Verification items for the finished model (mm, model axes). A direction names the side the tool comes from. Round coordinates to 2 decimals unless told otherwise and drop trailing zeros. Write each loop counter-clockwise with the first axis right and the second up, starting at its lowest first coordinate (ties: lowest second). Pieces come first, ordered by that corner, then holes. Notation, with made-up numbers: M 39,-5 L 85,-5 A30 cw 85,27 Z; hole C 61,41.5 d2. An arc over 180 degrees is marked long. One line per item, written item: value. Start each with the question number.
Item 1: Section check A-A, the plane y = 44. Record the cut outline in (x, z), then the cut area to 3 significant figures.
Item 2: Section check D-D, the plane x = 0.5. Record the cut outline in (y, z).
Item 3: Section check B-B, the plane x = 17.5. Record the cut outline in (y, z).
Item 4: Thickness scan on probe 1 along Z at (x, y) = (17.5, -17.25); probe 2 along X at (y, z) = (-18, 5.25); probe 3 along Z at (x, y) = (-9, 40). Record the ranges inside material, lowest first. Write a range as from..to.
Item 5: Draft check along X on faces 1 (the face through (17, -8, 2)), 2 (the face through (-15, -32, 2)), 3 (the face through (0, -2, 3.1)). Enter one of: +X half, -X half, draft (parallel to the pull), parting line (faces both ways), or undercut.
Item 6: Tool access check on faces 4 (the face through (-7, 35, 2)), 5 (the face through (18.655, -21.605, 2.021)), 6 (the face through (0, -2, 0)), 7 (the face through (-18, -8, 2)), 8 (the face through (15.85, 44, 2)). Record the directions out of +Z, -Z, +X, -X, +Y, -Y that give a thin tool (end or side, any length) a straight path to the whole face; none if there is none.
Item 7: Gauge pin test, flat ends, axial feed: pin 1 (0.9 mm diameter, centred on y = -11, z = 1.5, fed in from -X); pin 2 (2.5 mm diameter, centred on y = 46.5, z = 1.5, fed in from -X); pin 3 (1.6 mm diameter, centred on y = -10, z = 1, fed in from +X); pin 4 (2 mm diameter, centred on x = -17.5, z = 8.6, fed in from +Y). Record the tip position at first contact, or that the pin passes through.
Item 8: Section check C-C, the plane z = 8.6. Record the cut outline in (x, y), then the cut area to 3 significant figures.
from build123d import *

# Parameters (mm, degrees)
F0_W      = 3.95
F0_H      = 17.6
F0_W_2    = 3.8
F1_DEPTH  = 3.1
F2_W      = 40
F2_H      = 24
F3_DEPTH  = 1.5
F5_DEPTH  = 1.5
F6_W      = 5
F6_H      = 15
F7_DEPTH  = 8
F8_W      = 5
F8_H      = 6
F9_DEPTH  = 4.601
F10_R     = 1.25
F11_DEPTH = 15
F12_R     = 1.25
F13_DEPTH = 15


with BuildPart() as f1:
    # F0 (on Top) → F1 (new body)
    with BuildSketch(Plane.XY):
        with Locations((0.025, 43.8)):
            Rectangle(F0_W, F0_H)
        with Locations((-13.95, 43.8)):
            Rectangle(F0_W_2, F0_H)
        with Locations((13.95, 43.8)):
            Rectangle(F0_W_2, F0_H)
        Polygon((20, -35), (20, 35), (15.85, 35), (12.05, 35), (2, 35), (-1.95, 35), (-12.05, 35), (-15.85, 35), (-20, 35), (-20, -35), align=None)
    extrude(amount=F1_DEPTH)

    # F2 (on face) → F3 (join)
    with BuildSketch(Plane.XY.offset(3.1)):
        with Locations((0, 42)):
            Rectangle(F2_W, F2_H)
    extrude(amount=F3_DEPTH)

    # F4 (on face) → F5 (join)
    with BuildSketch(Plane(origin=(0, 0, 0), x_dir=(1, 0, 0), z_dir=(0, 0, -1))):
        Polygon((20.048024, -30), (20, -30), (20, -35), (15.85, -35), (15.85, -52.6), (12.05, -52.6), (12.05, -35), (2, -35), (2, -52.6), (-1.95, -52.6), (-1.95, -35), (-12.05, -35), (-12.05, -52.6), (-15.85, -52.6), (-15.85, -35), (-20, -35), (-20, -54), (20.048024, -54), align=None)
        Polygon((20, -30), (-20, -30), (-20, -35), (-15.85, -35), (-15.85, -52.6), (-12.05, -52.6), (-12.05, -35), (-1.95, -35), (-1.95, -52.6), (2, -52.6), (2, -35), (12.05, -35), (12.05, -52.6), (15.85, -52.6), (15.85, -35), (20, -35), align=None)
    extrude(amount=F5_DEPTH)

    # F6 (on face) → F7 (join)
    with BuildSketch(Plane.XY.offset(3.1)):
        with Locations((17.5, -21.5)):
            Rectangle(F6_W, F6_H)
        with Locations((-17.5, -21.5)):
            Rectangle(F6_W, F6_H)
    extrude(amount=F7_DEPTH)

    # F8 (on face) → F9 (cut, through all)
    with BuildSketch(Plane.XY.offset(3.1)):
        with Locations((17.5, -32)):
            Rectangle(F8_W, F8_H)
        with Locations((17.5, -11)):
            Rectangle(F8_W, F8_H)
        with Locations((-17.5, -11)):
            Rectangle(F8_W, F8_H)
        with Locations((-17.5, -32)):
            Rectangle(F8_W, F8_H)
    extrude(amount=-F9_DEPTH, mode=Mode.SUBTRACT)

    # F10 (on face) → F11 (cut, through all)
    with BuildSketch(Plane.XZ.offset(29)):
        with Locations((17.5, 8.6)):
            Circle(F10_R)
        with Locations((17.5, 2.5)):
            Circle(F10_R)
    extrude(amount=-F11_DEPTH, mode=Mode.SUBTRACT)

    # F12 (on face) → F13 (cut, through all)
    with BuildSketch(Plane.XZ.offset(29)):
        with Locations((-17.5, 8.6)):
            Circle(F12_R)
        with Locations((-17.5, 2.5)):
            Circle(F12_R)
    extrude(amount=-F13_DEPTH, mode=Mode.SUBTRACT)


solid = f1.part
Response values:
1. outline: M -20,-1.5 L 20.05,-1.5 L 20.05,0 L 15.85,0 L 15.85,3.1 L 20,3.1 L 20,4.6 L -20,4.6 L -20,3.1 L -15.85,3.1 L -15.85,0 L -20,0 Z; hole M -12.05,0 L -1.95,0 L -1.95,3.1 L -12.05,3.1 Z; hole M 2,0 L 12.05,0 L 12.05,3.1 L 2,3.1 Z
1. area: 156 mm2
2. outline: M -35,0 L 30,0 L 30,-1.5 L 54,-1.5 L 54,0 L 52.6,0 L 52.6,3.1 L 54,3.1 L 54,4.6 L 30,4.6 L 30,3.1 L -35,3.1 Z
3. outline: M -29,0 L -14,0 L -14,1.25 L -29,1.25 Z; M -29,3.75 L -14,3.75 L -14,7.35 L -29,7.35 Z; M -29,9.85 L -14,9.85 L -14,11.1 L -29,11.1 Z; M -8,0 L 30,0 L 30,-1.5 L 54,-1.5 L 54,0 L 35,0 L 35,3.1 L 54,3.1 L 54,4.6 L 30,4.6 L 30,3.1 L -8,3.1 Z
4. probe 1: z = 0..1.25, 3.75..7.35, 9.85..11.1
4. probe 2: x = -20..-15, 15..20
4. probe 3: z = -1.5..0, 3.1..4.6
5. face 1: draft
5. face 2: -X half
5. face 3: undercut
6. face 4: +Y
6. face 5: -Y
6. face 6: -Z, +X, -X, -Y
6. face 7: +Z, -Z, -X
6. face 8: +X, +Y
7. pin 1: stops at x = -15
7. pin 2: stops at x = -15.85
7. pin 3: stops at x = 15
7. pin 4: passes through
8. outline: M -20,-29 L -18.75,-29 L -18.75,-14 L -20,-14 Z; M -16.25,-29 L -15,-29 L -15,-14 L -16.25,-14 Z; M 15,-29 L 16.25,-29 L 16.25,-14 L 15,-14 Z; M 18.75,-29 L 20,-29 L 20,-14 L 18.75,-14 Z
8. area: 75.0 mm2
